Input: dimensioned drawing with shaded views. Units: mm. Origin: part minimum x, y, z. Give positions to 0.01 mm unless a question says otherwise; leave off trailing zeros. Loops run counter-clockwise (first coordinate to the right, second up) from the corner with the lowest first, then second, coordinate; pieces in that order, holes last. Notation, with made-up numbers: M 6,81 L 19,81 A19 cw 19,106 Z; hole C 44,-8.5 d8. An arc over 180 degrees is marked long. Use CSV: the item, a comma, the result in double quotes. Start each with the question number.
Q1. Section C-C, the plane x = 16. Output: boundary loops of the cut face in (y, z), plus the area to 3 significant figures.
Q2. Pin query (flat end, axial travel): pin 1 (1.5 mm diameter, centred on x = 67, y = 49, fed in from +Z). Return the tip coordinate at first contact, or that it passes through.
Q3. Material intervals for line 1 along Y through (x, z) = (152, 17.5); line 2 along X through (y, z) = (90.5, 18); line 3 along Z through (x, y) = (39.5, 69), sorted ascending.
Q4. Pull-direction query (X, two-part tool) for the marked faces 1, 2 and 3; classes: released by +X, released by -X, zero draft, split by the parting line, or undercut.
Q5. Section D-D, the plane x = 73. Output: boundary loops of the cut face in (y, z), plus the area to 3 significant figures.
Q6. Section B-B, the plane y = 26. Output: boundary loops of the cut face in (x, z).
Q7. Section A-A, the plane z = 17.75. Output: boundary loops of the cut face in (x, y), plus the area to 3 significant figures.
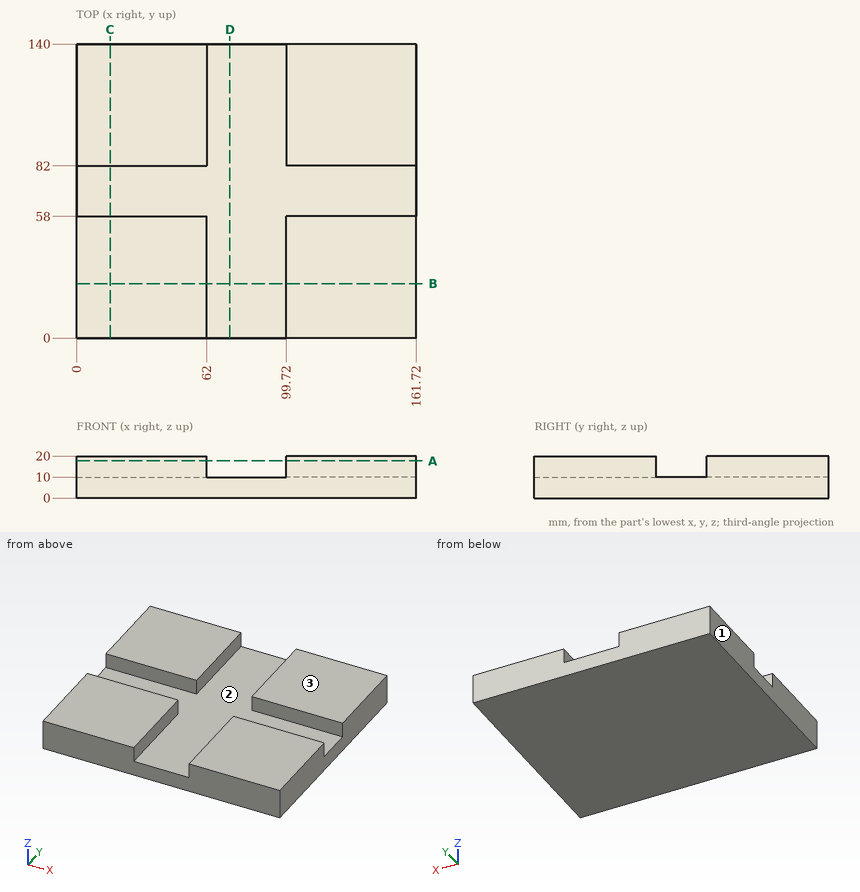
A:
1,outline,"M 0,0 L 140,0 L 140,20 L 82,20 L 82,10 L 58,10 L 58,20 L 0,20 Z"
1,area,"2,560 mm^2"
2,pin 1,"z = 10"
3,line 1,"0 to 58, 82 to 140"
3,line 2,"0 to 62, 99.72 to 161.72"
3,line 3,"0 to 10"
4,face 1,"released by -X"
4,face 2,"undercut"
4,face 3,"zero draft"
5,outline,"M 0,0 L 140,0 L 140,10 L 0,10 Z"
5,area,"1,400 mm^2"
6,outline,"M 0,0 L 161.72,0 L 161.72,20 L 99.72,20 L 99.72,10 L 62,10 L 62,20 L 0,20 Z"
7,outline,"M 0,0 L 62,0 L 62,58 L 0,58 Z; M 0,82 L 62,82 L 62,140 L 0,140 Z; M 99.72,0 L 161.72,0 L 161.72,58 L 99.72,58 Z; M 99.72,82 L 161.72,82 L 161.72,140 L 99.72,140 Z"
7,area,"14,400 mm^2"
